```python
from build123d import *

# Parameters (mm, degrees)
F0_W     = 101.6
F0_H     = 76.2
F1_DEPTH = 50.8
F4_D     = 25.4
F5_D     = 25.4
F6_W     = 22.86
F6_H     = 22.86
F7_DEPTH = 50.8
F8_SIZE  = 5.08


with BuildPart() as f1:
    # F0 (on Top) → F1 (new body)
    with BuildSketch(Plane.XY):
        Rectangle(F0_W, F0_H)
    extrude(amount=F1_DEPTH)

    # F4 (through all)
    with Locations(Plane(origin=(0, 38.1, 0), x_dir=(-1, 0, 0), z_dir=(0, 1, 0))):
        with Locations((-25.4, 25.4)):
            Hole(F4_D / 2)

    # F5 (through all)
    with Locations(Plane.XY.offset(50.8)):
        with Locations((25.4, 0)):
            Hole(F5_D / 2)

    # F6 (on face) → F7 (join)
    with BuildSketch(Plane.YZ.offset(50.8)):
        with Locations((0, 25.4)):
            Rectangle(F6_W, F6_H)
    extrude(amount=F7_DEPTH)

    # F8
    f8_edges = [f1.edges().sort_by_distance(p)[0] for p in [
        (50.8, 0, 50.8),
        (50.8, -38.1, 25.4),
        (50.8, 0, 0),
        (50.8, 38.1, 25.4),
    ]]
    chamfer(f8_edges, length=F8_SIZE)


solid = f1.part
```
The listing builds one solid part. Answer for the finished solid, in the listing's coordinates (mm). A direction names the side the tool comes from. Coordinates: 2 decimals unless noted, no trailing zeros. Loops run counter-clockwise (first coordinate to the right, second up) from the corner with the lowest first, then second, coordinate; pieces in that order, holes last. Notation, with made-up numbers: M 26.5,-35 L 65.5,-35 A17 ccw 65.5,-29 Z; hole C -16,4.5 d10. An arc over 180 degrees is marked long. Answer as a JSON object with one key per item and string values. Group by question number.
Item 1: Each of these flat-tipped pins is pushed along its axis until it touches: P1, Ø2, axis at x = 65.5, z = 15, coming from the -Y side; P2, Ø1, axis at x = 69.5, z = 30.5, coming from the +Y side; P3, Ø2, axis at y = 30, z = 14.5, coming from the +X side; P4, Ø15, axis at x = 25.4, z = 25.4, coming from the -Y side. Where does it stop, or does it pass through?
Item 2: Section C-C (y = 28.5) is taken. Write down the section's boundary in (x, z).
Item 3: Determine the mould class of faces 1 (the face through (76, 0, 13.97)), 2 (the face through (12.712, 23.017, 25.958)), 3 (the face through (101.6, 0, 26)), 4 (the face through (76, 0, 36.83)) for opening direction Z: +Z half, -Z half, draft (parallel to the pull), parting line (faces both ways), or undercut.
Item 4: Section A-A (y = 10) is taken. Write down the section's boundary in (x, z), and give its area (3 significant figures).
Item 5: Section B-B (z = 41.5) is taken. Write down the section's boundary in (x, y).
Item 6: Consider L1, parallel to X at y = -15, z = 25; L2, parallel to X at y = 0, z = 35.5; L3, parallel to Z at x = 25.4, y = 23. Determine where each line is inside the solid, lowest interval first.
Item 7: Which of the six approach directions +Z, -Z, +X, -X, +Y, -Y give full straight-line access (tool end or side, diameter ignored) to faces 5 (the face through (76, -11.43, 25)), 6 (the face through (-50.8, -1, 25)), 7 (the face through (76, 11.43, 25))?
Solved:
{
 "1": {"P1": "stops at y = -11.43", "P2": "stops at y = 11.43", "P3": "stops at x = 50.8", "P4": "passes through"},
 "2": {"outline": "M -50.8,0 L 45.72,0 L 50.8,5.08 L 50.8,45.72 L 45.72,50.8 L -50.8,50.8 Z; hole C 25.4,25.4 d25.4"},
 "3": {"face 1": "-Z half", "face 2": "undercut", "face 3": "draft", "face 4": "+Z half"},
 "4": {"outline": "M -50.8,0 L 17.57,0 L 17.57,15.4 A12.7 cw 17.57,35.4 L 17.57,50.8 L -50.8,50.8 Z; M 33.23,0 L 45.72,0 L 50.8,5.08 L 50.8,13.97 L 101.6,13.97 L 101.6,36.83 L 50.8,36.83 L 50.8,45.72 L 45.72,50.8 L 33.23,50.8 L 33.23,35.4 A12.7 cw 33.23,15.4 Z", "area": "5,370 mm2"},
 "5": {"outline": "M -50.8,-38.1 L 45.72,-38.1 L 50.8,-33.02 L 50.8,33.02 L 45.72,38.1 L -50.8,38.1 Z; hole C 25.4,0 d25.4"},
 "6": {"L1": "x = -50.8 to 12.71, 38.09 to 50.8", "L2": "x = -50.8 to 12.7, 38.1 to 101.6", "L3": "z = 0 to 12.7, 38.1 to 50.8"},
 "7": {"face 5": "+Z, -Z, +X, -Y", "face 6": "+Z, -Z, -X, +Y, -Y", "face 7": "+Z, -Z, +X, +Y"}
}
